Autodesk Inventor part; units mm, degrees
ref_plane "YZ Plane" through (0, 0, 0) normal (1, 0, 0) x (0, 1, 0)
ref_plane "XZ Plane" through (0, 0, 0) normal (0, 1, 0) x (-1, 0, 0)
ref_plane "XY Plane" through (0, 0, 0) normal (0, 0, 1) x (1, 0, 0)
sketch "Sketch1" plane through (0, 0, 0) normal (0, 0, 1) x (1, 0, 0)
  line L0 (0, 0) -> (80, 0)
  line L1 (80, 0) -> (80, 148.736)
  line L2 (80, 148.736) -> (0, 148.736)
  line L3 (0, 148.736) -> (0, 0)
  circle A0 centre (40, 93.486) radius 20
  circle A1 centre (16.75, 116.736) radius 4.5
  circle A2 centre (63.25, 116.736) radius 4.5
  circle A3 centre (16.75, 70.236) radius 4.5
  circle A4 centre (63.25, 70.236) radius 4.5
  dimension "d0" = 40
  dimension "d1" = 23.25
  dimension "d2" = 23.25
  dimension "d3" = 23.25
  dimension "d4" = 23.25
  dimension "d5" = 23.25
  dimension "d6" = 23.25
  dimension "d7" = 23.25
  dimension "d8" = 23.25
  dimension "d9" = 9
  dimension "d10" = 93.486
  dimension "d11" = 80
  dimension "d12" = 40
  dimension "d13" = 32
extrude "Extrusion1" add sketch "Sketch1" against normal blind 25
sketch "Sketch2" plane through (0, 0, 0) normal (0, 0, 1) x (1, 0, 0)
  circle A0 centre (16.75, 116.736) radius 4.5
  circle A1 centre (63.25, 116.736) radius 4.5
  circle A2 centre (16.75, 70.236) radius 4.5
  circle A3 centre (63.25, 70.236) radius 4.5
  circle A4 centre (16.75, 116.736) radius 8
  circle A5 centre (63.25, 116.736) radius 8
  circle A6 centre (16.75, 70.236) radius 8
  circle A7 centre (63.25, 70.236) radius 8
  point P0 (0, 0)
  dimension "d16" = 16
  dimension "d17" = 16
  dimension "d18" = 16
  dimension "d19" = 16
extrude "Extrusion2" cut sketch "Sketch2" against normal blind 8 contours A0 | A1 | A2 | A3 | A4 | A5 | A6 | A7
fillet "Fillet1" radius 2 4 edges at (80, 148.736, -12.5) (0, 148.736, -12.5) (80, 0, -12.5) (0, 0, -12.5)
sketch "Sketch3" plane through (2, 0, 0) normal (0, -1, 0) x (1, 0, 0)
  line L0 (-2, 0) -> (-2, -25)
  line L1 (78, -25) -> (78, 0)
  line L2 (0, 0) -> (76, 0)
  point P0 (20, -12.5)
  point P1 (56, -12.5)
  dimension "d28" = 22
  dimension "d29" = 12.5
  dimension "d30" = 22
  dimension "d31" = 12.5
hole "Hole1" at (58, 0, -12.5) at (22, 0, -12.5) direction (0, 1, 0) diameter 8.376 depth 25 tip angle 137
equation "\"d2\" = d1"
equation "\"d3\" = d1"
equation "\"d4\" = d1"
equation "\"d5\" = d1"
equation "\"d6\" = d1"
equation "\"d7\" = d1"
equation "\"d8\" = d1"
equation "\"d12\" = 0.5 * d11"
properties part number "Soporte1_CilindroHorizontal"
Verification items for the finished model (mm, model axes). A direction names the side the tool comes from. Give positions to 0.01 mm unless a question says otherwise; leave off trailing zeros. Loops run counter-clockwise (first coordinate to the right, second up) from the corner with the lowest first, then second, coordinate; pieces in that order, holes last.
1. Go/stop test with flat-tipped pins: P1, Ø8, axis at x = 15, y = 119, coming from the +Z side; P2, Ø5.5, axis at x = 16.75, y = 70.236, coming from the +Z side; P3, Ø1, axis at x = 22.5, z = -12, coming from the -Y side. Record where each tip stops, or that it passes through.
Derived:
P1: stops at z = -8
P2: passes through
P3: stops at y = 26.17
2. Tool access check on faces 3 (the cylindrical face through (16.164, 74.698, -16.381)), 4 (the flat face through (67, 113, -8)), 5 (the cylindrical face through (20.742, 12.675, -16.495)). Record the directions out of +Z, -Z, +X, -X, +Y, -Y that give a thin tool (end or side, any length) a straight path to the whole face; none if there is none.
Derived:
face 3: +Z, -Z
face 4: +Z
face 5: -Y
3. Cross-section at A-A on x = 40. Record the cut outline in (y, z), and give its area (3 significant figures).
Derived:
outline: (0, -25) - (73.49, -25) - (73.49, 0) - (0, 0) - close; (113.49, -25) - (148.74, -25) - (148.74, 0) - (113.49, 0) - close
area: 2,720 mm2
4. Release check for a two-part mould opening along X. For faces 1 (the flat face through (31, 75, 0)), 2 (the cylindrical face through (62.21, 124.67, -3.94)) record: +X half, -X half, draft (parallel to the pull), parting line (faces both ways), or undercut.
Derived:
face 1: draft
face 2: undercut
5. Cross-section at D-D on z = -22.75. Record the cut outline in (x, y).
Derived:
outline: (0, 2) arc R2 ccw to (2, 0) - (78, 0) arc R2 ccw to (80, 2) - (80, 146.74) arc R2 ccw to (78, 148.74) - (2, 148.74) arc R2 ccw to (0, 146.74) - close; hole circle Ø9 at (16.75, 70.24); hole circle Ø9 at (16.75, 116.74); hole circle Ø40 at (40, 93.49); hole circle Ø9 at (63.25, 70.24); hole circle Ø9 at (63.25, 116.74)
6. Cross-section at B-B on z = -3.25. Record the cut outline in (x, y).
Derived:
outline: (0, 2) arc R2 ccw to (2, 0) - (78, 0) arc R2 ccw to (80, 2) - (80, 146.74) arc R2 ccw to (78, 148.74) - (2, 148.74) arc R2 ccw to (0, 146.74) - close; hole circle Ø16 at (16.75, 70.24); hole circle Ø16 at (16.75, 116.74); hole circle Ø40 at (40, 93.49); hole circle Ø16 at (63.25, 70.24); hole circle Ø16 at (63.25, 116.74)
7. Cross-section at C-C on y = 105.5. Record the cut outline in (x, z), and give its area (3 significant figures).
Derived:
outline: (0, -25) - (24.01, -25) - (24.01, 0) - (0, 0) - close; (55.99, -25) - (80, -25) - (80, 0) - (55.99, 0) - close
area: 1,200 mm2
8. Material ranges on probe 1 along X at (y, z) = (19.25, -12.5); probe 2 along Y at (x, z) = (63.25, -2.25); probe 3 along X at (y, z) = (123, -5.25), recorded low to high.
Derived:
probe 1: x = 0 to 17.81, 26.19 to 53.81, 62.19 to 80
probe 2: y = 0 to 62.24, 78.24 to 108.74, 124.74 to 148.74
probe 3: x = 0 to 11.77, 21.73 to 58.27, 68.23 to 80
